Autodesk Inventor part; units mm, degrees
ref_plane "Work Plane1" through (0, 0, -15) normal (0, 0, 1) x (1, 0, 0)
ref_plane "YZ Plane" through (0, 0, 0) normal (1, 0, 0) x (0, 1, 0)
ref_plane "XZ Plane" through (0, 0, 0) normal (0, 1, 0) x (-1, 0, 0)
sketch "Sketch1" plane through (0, 0, 0) normal (0, 0, 1) x (1, 0, 0)
  line L0 (0, 0) -> (25, 0)
  line L1 (25, 0) -> (25, 40)
  line L2 (25, 40) -> (0, 40)
  line L3 (0, 40) -> (0, 0)
  dimension "d1" = 25
  dimension "d2" = 40
  dimension "d3" = 25
extrude "Extrusion1" add sketch "Sketch1" against normal blind 30
sketch "Sketch2" plane through (25, 0, 0) normal (1, 0, 0) x (0, 0, -1)
  line L0 (0, 0) -> (30, 0)
  circle A0 centre (15, 6.56) radius 2.46
extrude "Extrusion2" cut sketch "Sketch2" against normal blind 30
sketch "Sketch3" plane through (0, 0, 0) normal (-1, 0, 0) x (0, 0, 1)
  line L0 (0, 0) -> (-30, 0)
  line L1 (-25.05, 0) -> (-4.95, 0)
  line L2 (-4.95, 0) -> (-4.95, 33.12)
  line L3 (-4.95, 33.12) -> (-25.05, 33.12)
  line L4 (-25.05, 33.12) -> (-25.05, 0)
  dimension "d11" = 20.1
extrude "Extrusion3" cut sketch "Sketch3" against normal blind 20
sketch "Sketch4" plane through (0, 0, 0) normal (0, -1, 0) x (1, 0, 0)
  line L0 (20, -4.95) -> (20, -25.05)
  line L1 (20, -15) -> (25, -15)
  line L2 (25, 0) -> (25, -30)
  line L3 (20, -8.025) -> (25, -8.025)
  line L4 (25, -8.025) -> (25, -21.975)
  line L5 (25, -21.975) -> (20, -21.975)
  line L6 (20, -21.975) -> (20, -8.025)
  line L7 (20, -8.025) -> (25, -21.975) construction
  line L8 (25, -8.025) -> (20, -21.975) construction
  line L9 (25, -12.54) -> (25, -17.46)
  point P0 (0, 0)
  point P1 (22.5, -15)
  dimension "d14" = 13.95
extrude "Extrusion4" add sketch "Sketch4" along normal blind 15
sketch "Sketch5" plane through (20, 0, 0) normal (-1, 0, 0) x (0, 0, 1)
  circle A0 centre (-15, 6.56) radius 2.46
  circle A1 centre (-15, 6.56) radius 4.7025
  circle A2 centre (-15, 6.56) radius 2.46
  circle A3 centre (-15, 6.56) radius 2.46
  point P0 (0, 0)
  dimension "d17" = 9.405
extrude "Extrusion5" cut sketch "Sketch5" against normal blind 2.1
sketch "Sketch6" plane through (25, 0, 0) normal (1, 0, 0) x (0, 0, -1)
  circle A0 centre (15, 6.56) radius 4.7025
  line L0 (15, 6.56) -> (15, 23.56)
  circle A1 centre (15, 23.56) radius 2.46
  point P0 (0, 0)
  dimension "d20" = 17
  dimension "d21" = 4.92
extrude "Extrusion6" cut sketch "Sketch6" against normal blind 10 contours A1
sketch "Sketch7" plane through (20, 0, 0) normal (-1, 0, 0) x (0, 0, 1)
  circle A0 centre (-15, 23.56) radius 2.46
  circle A1 centre (-15, 23.56) radius 4.7025
  point P0 (0, 0)
  dimension "d24" = 9.405
extrude "Extrusion7" cut sketch "Sketch7" against normal blind 2.1
sketch "Sketch9" plane through (25, 0, 0) normal (1, 0, 0) x (0, 0, -1)
  circle A0 centre (15, 6.56) radius 2.46
  circle A1 centre (15, 6.56) radius 2.46
  circle A2 centre (15, 23.56) radius 2.46
  circle A3 centre (15, 23.56) radius 2.46
  line L0 (30, 40) -> (30, 0)
  line L1 (30, 0) -> (30, 40)
  line L2 (30, 40) -> (0, 40)
  line L3 (0, 40) -> (0, 0)
  line L4 (0, 0) -> (8.025, 0)
  line L5 (21.975, 0) -> (21.975, -15)
  line L6 (21.975, -15) -> (8.025, -15)
  line L7 (8.025, -15) -> (8.025, 0)
  line L8 (0, 0) -> (8.025, 0)
  line L9 (21.975, 0) -> (30, 0)
extrude "Extrusion8" add sketch "Sketch9" along normal blind 5
sketch "Sketch10" plane through (0, 40, 0) normal (0, 1, 0) x (1, 0, 0)
  line L0 (0, 30) -> (30, 30)
  line L1 (30, 0) -> (0, 0)
  line L2 (0, 30) -> (30, 30)
  line L3 (30, 30) -> (30, 0)
  line L4 (30, 0) -> (0, 0)
  line L5 (0, 0) -> (0, 30)
extrude "Extrusion9" add sketch "Sketch10" along normal blind 30
sketch "Sketch12" plane through (30, 0, 0) normal (1, 0, 0) x (0, 0, -1)
  circle A0 centre (15, 6.56) radius 2.46
  line L0 (15, 6.56) -> (15, 15.06)
  circle A1 centre (15, 15.06) radius 2.525
  point P0 (0, 0)
  dimension "d31" = 8.5
  dimension "d33" = 5.05
extrude "Extrusion10" cut sketch "Sketch12" against normal blind 30 contours A1
sketch "Sketch14" plane through (0, 0, 0) normal (0, 0, 1) x (1, 0, 0)
  line L0 (30, 70) -> (0, 70)
  line L1 (0, 100) -> (-8, 100)
  line L2 (30, 0) -> (30, 70)
  line L3 (30, 118) -> (30, 70)
  line L4 (30, 105) -> (30, 100)
  line L5 (-2, 134) -> (-8, 136)
  line L6 (-2, 134) -> (4, 118)
  line L7 (-2, 102) -> (-8, 100)
  line L8 (-2, 102) -> (4, 118)
  line L9 (0, 70) -> (30, 70)
  line L10 (0, 70) -> (0, 100)
  line L11 (15, 136) -> (30, 118)
  line L12 (-8, 136) -> (15, 136)
  point P0 (0, 0)
  dimension "d47" = 30
extrude "Extrusion12" add sketch "Sketch14" against normal blind 30
sketch "Sketch15" plane through (0, 0, -25.05) normal (-1, 0, 0) x (0, 0, 1)
  line L0 (0, 33.12) -> (20.1, 33.12)
  line L1 (20.1, 33.12) -> (20.1, 0)
  line L2 (0, 33.12) -> (20.1, 33.12)
  line L3 (20.1, 33.12) -> (20.1, 31.1)
  line L4 (20.1, 31.1) -> (0, 31.1)
  line L5 (0, 31.1) -> (0, 33.12)
  point P0 (25.05, 0)
  dimension "d57" = 2.02
extrude "Extrusion13" add sketch "Sketch15" against normal blind 20
sketch "Sketch23" plane through (0, 0, 0) normal (0, 0, 1) x (1, 0, 0)
  line L0 (0, 100) -> (-8, 100)
  line L1 (-8, 100) -> (-2, 102)
  line L2 (-8, 100) -> (-2, 102)
  line L3 (-2, 102) -> (4, 118)
  line L4 (-2, 102) -> (4, 118)
  line L5 (-2, 134) -> (4, 118)
  line L6 (4, 118) -> (-2, 134)
  line L7 (-2, 134) -> (-8, 136)
  line L8 (-2, 134) -> (-8, 136)
  line L9 (-8, 136) -> (15, 136)
  line L10 (-8, 136) -> (15, 136)
  line L11 (30, 118) -> (15, 136)
  line L12 (15, 136) -> (30, 118)
  line L13 (30, 118) -> (30, 93)
  line L14 (30, 0) -> (30, 118)
  line L15 (30, 93) -> (0, 93)
  line L16 (0, 93) -> (0, 100)
  line L17 (-8, 100) -> (0, 100)
  point P0 (0, 0)
  dimension "d85" = 25
extrude "Extrusion14" add sketch "Sketch23" along normal blind 45
ref_plane "Work Plane1" through (0, 0, -15) normal (0, 0, 1) x (1, 0, 0)
mirror "Mirror1" about plane through (0, 0, -15) normal (0, 0, 1) of "Extrusion14"
properties part number "32mm_x_120mm"
Part model, mm, in its own coordinate system. A direction names the side the tool comes from. Coordinates: 2 decimals unless noted, no trailing zeros. Order: outer loops, then holes, each group sorted by start corner. A loop starts at its lowest first (then second) coordinate and runs counter-clockwise, first axis right, second up. Notation, with made-up numbers: (-27.5, 42.5) - (27.5, 42.5) arc R12 ccw to (27.5, 57.5) - close; hole circle Ø10 at (81, -25). An arc over 180 degrees is marked (long way). Return JSON: item names as keys, results as strings. Group by question number.
Item 1: Pull direction Z, two halves, no side cores. Call faces 1 (the face through (30, 65, -14)), 2 (the face through (15, 47, -30)), 3 (the face through (20, 8, -20)): pulls with the +Z half, pulls with the -Z half, needs draft (parallel to the pull), parting line crosses it, or undercut.
Item 2: Which spindle directions (+Z, -Z, +X, -X, +Y, -Y) get a long thin tool onto all of the face, cutting with end or side? Do faces 4 (the face through (25, -8, -8.025)), 5 (the face through (0, 62, -14)), 6 (the face through (10, 31.1, -15)), 7 (the face through (-5, 101, -14)), 8 (the face through (25, -7, -21.975)). Say none if no direction does.
Item 3: Cut at A-A (y = 6.56). List the corners of the cut face in (x, z), plus the area to 3 significant figures.
Item 4: Cut at D-D (x = 17.5). List the corners of the cut face in (y, z), plus the area to 3 significant figures.
Item 5: Pin check, flat tips, straight feed: pin 1 (5.5 mm diameter, centred on y = 6.56, z = -15, fed in from -X); pin 2 (2.5 mm diameter, centred on x = -4.5, z = -16, fed in from -Y); pin 3 (6 mm diameter, centred on x = 17.5, y = 52, fed in from +Z); pin 4 (8 mm diameter, centred on x = 24.5, y = 90.5, fed in from +Z). Stop position of each tip, or through.
Item 6: Cut at C-C (z = -66). List the corners of the cut face in (x, y), plus the area to 3 significant figures.
Item 7: Cut at B-B (z = -15). State how many separate pieces and enclosed holes the cut face has, plus the area to 3 significant figures.
Item 8: Drill centre lines: probe 1 along Z at (x, y) = (27.5, 23.56); probe 2 along Y at (x, z) = (27, -15) (3 decimals); probe 3 along X at (y, z) = (8.5, -13). Where is each one in solid material? Low to high. Write a range as from..to.
Check values:
{
 "1": {"face 1": "needs draft", "face 2": "pulls with the -Z half", "face 3": "undercut"},
 "2": {"face 4": "+Z, +X, -X, -Y", "face 5": "+Z, -Z, -X, -Y", "face 6": "-X, -Y", "face 7": "+Z, -Z, -X", "face 8": "-Z, +X, -X, -Y"},
 "3": {"outline": "(0, -30) - (30, -30) - (30, -17.46) - (22.1, -17.46) - (22.1, -19.7) - (20, -19.7) - (20, -25.05) - (0, -25.05) - close; (0, -4.95) - (20, -4.95) - (20, -10.3) - (22.1, -10.3) - (22.1, -12.54) - (30, -12.54) - (30, 0) - (0, 0) - close", "area": "439 mm2"},
 "4": {"outline": "(0, -30) - (93, -30) - (93, -75) - (133, -75) - (133, 45) - (93, 45) - (93, 0) - (0, 0) - (0, -4.95) - (31.1, -4.95) - (31.1, -25.05) - (0, -25.05) - close", "area": "6,960 mm2"},
 "5": {"pin 1": "stops at x = 22.1", "pin 2": "stops at y = 100", "pin 3": "stops at z = 0", "pin 4": "stops at z = 45"},
 "6": {"outline": "(-8, 100) - (0, 100) - (0, 93) - (30, 93) - (30, 118) - (15, 136) - (-8, 136) - (-2, 134) - (4, 118) - (-2, 102) - close", "area": "1,140 mm2"},
 "7": {"separate pieces": "4", "enclosed holes": "0", "area": "3,290 mm2"},
 "8": {"probe 1": "z = -30..-17.46, -12.54..0", "probe 2": "y = -15..4.1, 9.02..12.535, 17.585..21.1, 26.02..121.6", "probe 3": "x = 22.1..30"}
}
